Design review of the part built by this model. Coordinates are the model's own, in mm. A direction names the side the tool comes from. Coordinates: 2 decimals unless noted, no trailing zeros. Write each loop counter-clockwise with the first axis right and the second up, starting at its lowest first coordinate (ties: lowest second). Pieces come first, ordered by that corner, then holes.
Q1. For probe 1 along Y at (x, z) = (0, 0.95); probe 2 along Y at (x, z) = (14, 1.9) (3 decimals); probe 3 along Y at (x, z) = (9.5, 2.45) (3 decimals), list the stretches that pass through material, from the lowest coordinate up.
Q2. Take a section at C-C (z = 0.95). Give the boundary of the cut face in (x, y) (3 decimals).
Q3. Take a section at D-D (y = 13). Give the boundary of the cut face in (x, z) (3 decimals).
Q4. Mouldability with a two-part tool opening along Y and no side actions: class faces 1 (the flat face through (12.7, -9, 2)), 2 (the flat face through (14, -3.175, 2)), 3 (the cylindrical face through (-3.05, -1.26, 1.57)) as pulls with the +Y half, pulls with the -Y half, needs draft (parallel to the pull), parting line crosses it, or undercut.
Q5. Insertion check: pin 1 (1.6 mm diameter, centred on y = -10.5, z = 2, fed in from +X); pin 2 (4 mm diameter, centred on x = 0, y = 0, fed in from +Z); pin 3 (1 mm diameter, centred on y = -17, z = 1.5, fed in from -X) (3 decimals); pin 4 (1 mm diameter, centred on y = 3.5, z = 2.5, fed in from -X) (3 decimals). Each pin has a flat end and moves straight along its axis. Give the tip position at first contact, or say it passes through.
Q6. Machinability: for faces 4 (the flat face through (-14, 3.175, 2)), 5 (the flat face through (-12.7, -9, 2)), 6 (the flat face through (3.175, -16, 2)), which of the approach directions +Z, -Z, +X, -X, +Y, -Y give a long, thin tool a straight path to every point of the face, cutting with its end or side? Answer none if there is none.
Q7. Take a section at B-B (y = 0). Give the boundary of the cut face in (x, z) (3 decimals), and give its area (3 significant figures).
Q8. Take a section at A-A (x = 0). Give the boundary of the cut face in (y, z) (3 decimals), and give its area (3 significant figures).
```python
from build123d import *

# Parameters (mm, degrees)
EXTRUDE1_DEPTH     = 3.175
SKETCH2_R          = 3.302
CUT_EXTRUDE1_DEPTH = 3.175


with BuildPart() as part:
    # Sketch1 → Extrude1 (new body)
    with BuildSketch(Plane.XY):
        Polygon((-12.7, 14.605), (-3.175, 14.605), (-3.175, 17.78), (3.175, 17.78), (3.175, 14.605), (12.7, 14.605), (12.7, 3.175), (15.875, 3.175), (15.875, -3.175), (12.7, -3.175), (12.7, -14.605), (3.175, -14.605), (3.175, -17.78), (-3.175, -17.78), (-3.175, -14.605), (-12.7, -14.605), (-12.7, -3.175), (-15.875, -3.175), (-15.875, 3.175), (-12.7, 3.175), align=None)
    extrude(amount=EXTRUDE1_DEPTH)

    # Sketch2 → Cut-Extrude1 (cut)
    with BuildSketch(Plane(origin=(0, 0, 0), x_dir=(-1, 0, 0), z_dir=(0, 0, -1))):
        Circle(SKETCH2_R)
    extrude(amount=-CUT_EXTRUDE1_DEPTH, mode=Mode.SUBTRACT)


solid = part.part
```
Response:
1. probe 1: y = -17.78 to -3.3, 3.3 to 17.78
1. probe 2: y = -3.175 to 3.175
1. probe 3: y = -14.605 to 14.605
2. outline: (-15.875, -3.175) - (-12.7, -3.175) - (-12.7, -14.605) - (-3.175, -14.605) - (-3.175, -17.78) - (3.175, -17.78) - (3.175, -14.605) - (12.7, -14.605) - (12.7, -3.175) - (15.875, -3.175) - (15.875, 3.175) - (12.7, 3.175) - (12.7, 14.605) - (3.175, 14.605) - (3.175, 17.78) - (-3.175, 17.78) - (-3.175, 14.605) - (-12.7, 14.605) - (-12.7, 3.175) - (-15.875, 3.175) - close; hole circle Ø6.604 at (0, 0)
3. outline: (-12.7, 0) - (12.7, 0) - (12.7, 3.175) - (-12.7, 3.175) - close
4. face 1: needs draft
4. face 2: pulls with the -Y half
4. face 3: undercut
5. pin 1: stops at x = 12.7
5. pin 2: passes through
5. pin 3: stops at x = -3.175
5. pin 4: stops at x = -15.875
6. face 4: +Z, -Z, -X, +Y
6. face 5: +Z, -Z, -X, -Y
6. face 6: +Z, -Z, +X, -Y
7. outline: (-15.875, 0) - (-3.302, 0) - (-3.302, 3.175) - (-15.875, 3.175) - close; (3.302, 0) - (15.875, 0) - (15.875, 3.175) - (3.302, 3.175) - close
7. area: 79.8 mm2
8. outline: (-17.78, 0) - (-3.302, 0) - (-3.302, 3.175) - (-17.78, 3.175) - close; (3.302, 0) - (17.78, 0) - (17.78, 3.175) - (3.302, 3.175) - close
8. area: 91.9 mm2
